CAD build for the part. Positions are in the model's coordinates, mm. Give positions to 0.01 mm unless a question says otherwise; leave off trailing zeros. Order: outer loops, then holes, each group sorted by start corner. A loop starts at its lowest first (then second) coordinate and runs counter-clockwise, first axis right, second up.
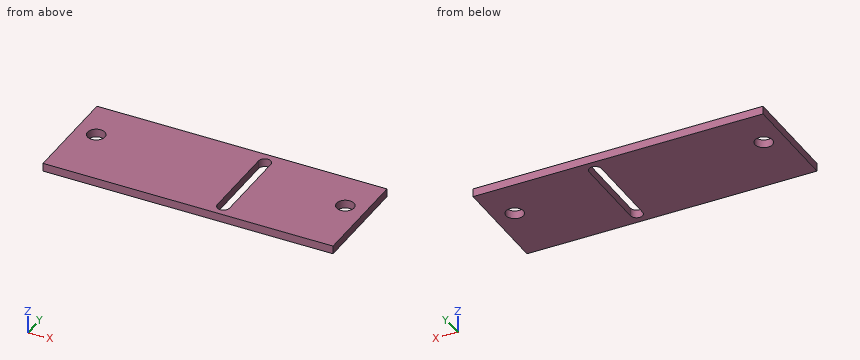
Autodesk Inventor part; units mm, degrees
ref_plane "YZ Plane" through (0, 0, 0) normal (1, 0, 0) x (0, 1, 0)
ref_plane "XZ Plane" through (0, 0, 0) normal (0, 1, 0) x (-1, 0, 0)
ref_plane "XY Plane" through (0, 0, 0) normal (0, 0, 1) x (1, 0, 0)
sketch "Sketch1" plane through (0, 0, 0) normal (0, 0, 1) x (1, 0, 0)
  line L0 (0, -6.35) -> (25.4, -6.35)
  line L1 (25.4, -6.35) -> (25.4, -31.75)
  line L2 (25.4, -31.75) -> (-25.4, -31.75)
  line L3 (-25.4, -31.75) -> (-25.4, -6.35)
  line L4 (-25.4, -6.35) -> (0, -6.35)
  point P0 (-6.35, -6.35)
  point P1 (6.35, -6.35)
  dimension "d7" = 25.4
  dimension "d8" = 25.4
  dimension "d9" = 50.8
extrude "Extrusion1" add sketch "Sketch1" along normal blind 2
sketch "Sketch2" plane through (0, 0, 2) normal (0, 0, 1) x (1, 0, 0)
  line L0 (-25.4, -6.35) -> (-25.4, -31.75)
  line L1 (-25.4, -31.75) -> (7.1, -31.75)
  line L2 (-25.4, -31.75) -> (25.4, -31.75)
  line L3 (7.1, -31.75) -> (7.1, -30.75)
  line L4 (7.1, -30.75) -> (7.1, -28.75)
  circle A0 centre (7.1, -28.75) radius 1.5
  circle A1 centre (7.1, -9.35) radius 1.5
  line L5 (5.6, -9.35) -> (5.6, -28.75)
  line L6 (8.6, -9.35) -> (8.6, -28.75)
  point P0 (0, 0)
  dimension "d10" = 32.5
  dimension "d11" = 1
  dimension "d12" = 2
  dimension "d13" = 3
  dimension "d15" = 3
extrude "Extrusion2" cut sketch "Sketch2" against normal blind 2.54
sketch "Sketch4" plane through (0, 0, 2) normal (0, 0, 1) x (1, 0, 0)
  line L0 (25.4, -6.35) -> (35.4, -6.35)
  line L1 (35.4, -6.35) -> (35.4, -16.35)
  circle A0 centre (30.4, -16.35) radius 2.125
  line L2 (25.4, -6.35) -> (35.4, -6.35)
  line L3 (35.4, -6.35) -> (35.4, -31.75)
  line L4 (35.4, -31.75) -> (25.4, -31.75)
  line L5 (25.4, -31.75) -> (25.4, -6.35)
  line L6 (25.4, -6.35) -> (-25.4, -6.35)
  line L7 (25.4, -6.35) -> (0, -6.35)
  line L8 (0, -6.35) -> (0, -31.75)
  line L9 (-25.4, -6.35) -> (-35.4, -6.35)
  line L10 (-35.4, -6.35) -> (-35.4, -16.35)
  circle A1 centre (-30.4, -16.35) radius 2.125
  line L11 (-25.4, -6.35) -> (-35.4, -6.35)
  line L12 (-35.4, -6.35) -> (-35.4, -31.75)
  line L13 (-35.4, -31.75) -> (-25.4, -31.75)
  line L14 (-25.4, -31.75) -> (-25.4, -6.35)
  point P0 (0, 0)
  dimension "d40" = 10
  dimension "d41" = 10
  dimension "d42" = 4.25
  dimension "d43" = 25.4
extrude "Extrusion4" add sketch "Sketch4" against normal blind 2
properties part number "Ultrasonic Sensor 2.0"
Item 1: Wall check: L1, parallel to X at y = -12, z = 1.15; L2, parallel to Y at x = 30.4, z = 0.8 (3 decimals); L3, parallel to X at y = -18, z = 0.7. Give the ranges that are in metal, low to high.
Item 2: Slice it at C-C (y = -22). Give the cut face in (x, z), and give its area (3 significant figures).
Item 3: Slice it at A-A (y = -16.35). Give the cut face in (x, z) (3 decimals).
Item 4: Slice it at D-D (x = -30.4). Give the cut face in (y, z) (3 decimals), and give its area (3 significant figures).
Item 5: Slice it at B-B (z = 0.5). Give the cut face in (x, y) (3 decimals).
A:
1. L1: x = -35.4 to 5.6, 8.6 to 35.4
1. L2: y = -31.75 to -18.475, -14.225 to -6.35
1. L3: x = -35.4 to -31.74, -29.06 to 5.6, 8.6 to 29.06, 31.74 to 35.4
2. outline: (-35.4, 0) - (5.6, 0) - (5.6, 2) - (-35.4, 2) - close; (8.6, 0) - (35.4, 0) - (35.4, 2) - (8.6, 2) - close
2. area: 136 mm2
3. outline: (-35.4, 0) - (-32.525, 0) - (-32.525, 2) - (-35.4, 2) - close; (-28.275, 0) - (5.6, 0) - (5.6, 2) - (-28.275, 2) - close; (8.6, 0) - (28.275, 0) - (28.275, 2) - (8.6, 2) - close; (32.525, 0) - (35.4, 0) - (35.4, 2) - (32.525, 2) - close
4. outline: (-31.75, 0) - (-18.475, 0) - (-18.475, 2) - (-31.75, 2) - close; (-14.225, 0) - (-6.35, 0) - (-6.35, 2) - (-14.225, 2) - close
4. area: 42.3 mm2
5. outline: (-35.4, -31.75) - (35.4, -31.75) - (35.4, -6.35) - (-35.4, -6.35) - close; hole circle Ø4.25 at (-30.4, -16.35); hole (5.6, -28.75) arc R1.5 ccw to (8.6, -28.75) - (8.6, -9.35) arc R1.5 ccw to (5.6, -9.35) - close; hole circle Ø4.25 at (30.4, -16.35)
